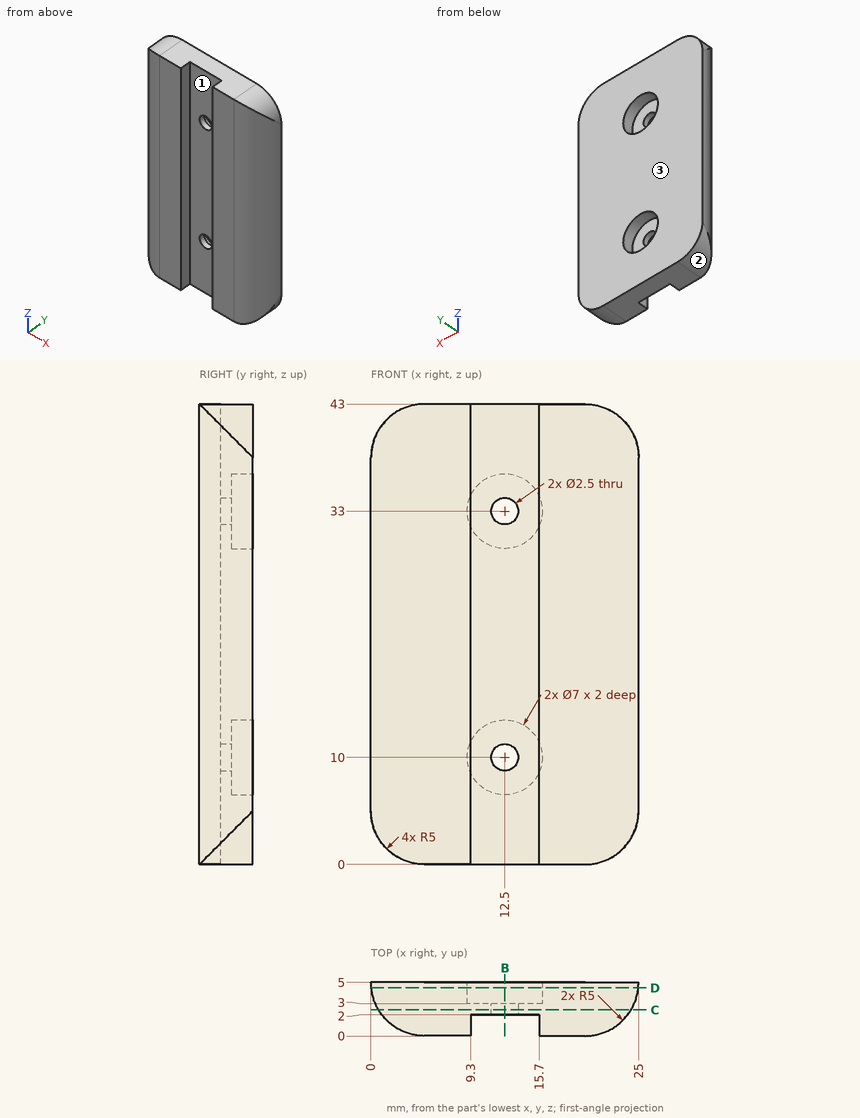
Job drawing, mm, ordinate dimensions from the low corner. One solid piece. Coordinates: 2 decimals unless noted, no trailing zeros. Loops run counter-clockwise (first coordinate to the right, second up) from the corner with the lowest first, then second, coordinate; pieces in that order, holes last. Notation, with made-up numbers: (21, 62) -> (54, 62) arc R25 cw to (54, 81) -> close; hole circle Ø5 at (-21, 39). An arc over 180 degrees is marked (long way). One line per item, written item: value.
1. Flat gauge pins, fed straight in: P1, Ø4, axis at x = 12.5, z = 10, coming from the -Y side; P2, Ø7.5, axis at x = 13.5, z = 10, coming from the +Y side; P3, Ø1.6, axis at y = 0.5, z = 13, coming from the -X side (1 decimal); P4, Ø2, axis at x = 14, z = 33.5, coming from the +Y side. Where does each tip first touch, or does it go through?
Answers:
P1: stops at y = 2
P2: stops at y = 5
P3: stops at x = 1.6
P4: stops at y = 3
2. Slice it at C-C on y = 2.45. Write the cut outline in (x, z).
Answers:
outline: (0.7, 2.45) arc R5 ccw to (5, 0) -> (20, 0) arc R5 ccw to (24.3, 2.45) -> (24.3, 40.55) arc R5 ccw to (20, 43) -> (5, 43) arc R5 ccw to (0.7, 40.55) -> close; hole circle Ø2.5 at (12.5, 10); hole circle Ø2.5 at (12.5, 33)
3. Slice it at D-D on y = 4.5. Write the cut outline in (x, z) (1 decimal), and give its area (3 significant figures).
Answers:
outline: (0, 4.5) arc R5 ccw to (5, 0) -> (20, 0) arc R5 ccw to (25, 4.5) -> (25, 38.5) arc R5 ccw to (20, 43) -> (5, 43) arc R5 ccw to (0, 38.5) -> close; hole circle Ø7 at (12.5, 10); hole circle Ø7 at (12.5, 33)
area: 975 mm^2
4. Pull direction X, two halves, no side cores. Call the marked faces 1, 2 and 3: pulls with the +X half, pulls with the -X half, needs draft (parallel to the pull), parting line crosses it, or undercut.
Answers:
face 1: undercut
face 2: pulls with the -X half
face 3: needs draft
5. Slice it at B-B on x = 12.5. Write the cut outline in (y, z).
Answers:
outline: (2, 0) -> (5, 0) -> (5, 6.5) -> (3, 6.5) -> (3, 8.75) -> (2, 8.75) -> close; (2, 11.25) -> (3, 11.25) -> (3, 13.5) -> (5, 13.5) -> (5, 29.5) -> (3, 29.5) -> (3, 31.75) -> (2, 31.75) -> close; (2, 34.25) -> (3, 34.25) -> (3, 36.5) -> (5, 36.5) -> (5, 43) -> (2, 43) -> close
6. Drill centre lines: line 1 (Z direction, x = 12.5, y = 2.6); line 2 (X direction, y = 4.85, z = 17.5); line 3 (Y direction, x = 12.5, z = 3). Where is each one in solid material? Low to high. Write a range as [from, to].
Answers:
line 1: z = [0, 8.75], [11.25, 31.75], [34.25, 43]
line 2: x = [0, 25]
line 3: y = [2, 5]
